For this review, take the finished solid that the model builds, in its own axes (mm). A direction names the side the tool comes from. Give positions to 0.01 mm unless a question says otherwise; leave off trailing zeros. Loops run counter-clockwise (first coordinate to the right, second up) from the corner with the lowest first, then second, coordinate; pieces in that order, holes last.
```python
from build123d import *

# Parameters (mm, degrees)
SKETCH_1_R          = 11
SKETCH_1_R_2        = 1
EXTRUDE_1_DEPTH     = 4
EXTRUDE_START       = -12
SKETCH_3_R          = 1
EXTRUDE_2_DEPTH     = 12
SKETCH_12_R         = 1
CUT_EXTRUDE_4_DEPTH = 20
SKETCH_13_R         = 7.5
CUT_EXTRUDE_5_DEPTH = 17.062378404
EXTRUDE_START_2     = -1
SKETCH_14_R         = 1
EXTRUDE_3_DEPTH     = 1
CHAMFER_1_SIZE      = 0.2


with BuildPart() as part:
    # 草图1 → 凸台-拉伸1 (new body)
    with BuildSketch(Plane.XY):
        Circle(SKETCH_1_R)
        with Locations((9, 0)):
            Circle(SKETCH_1_R_2, mode=Mode.SUBTRACT)
        with Locations((2.781152949, -8.559508647)):
            Circle(SKETCH_1_R_2, mode=Mode.SUBTRACT)
        with Locations((-7.281152949, -5.290067271)):
            Circle(SKETCH_1_R_2, mode=Mode.SUBTRACT)
        with Locations((-7.281152949, 5.290067271)):
            Circle(SKETCH_1_R_2, mode=Mode.SUBTRACT)
        with Locations((2.781152949, 8.559508647)):
            Circle(SKETCH_1_R_2, mode=Mode.SUBTRACT)
    extrude(amount=EXTRUDE_1_DEPTH)

    # 草图3 → 凸台-拉伸2 (add)
    with BuildSketch(Plane.XY.offset(4).offset(EXTRUDE_START)):
        with Locations((9, 0)):
            Circle(SKETCH_3_R)
        with Locations((2.781152949, -8.559508647)):
            Circle(SKETCH_3_R)
        with Locations((-7.281152949, -5.290067271)):
            Circle(SKETCH_3_R)
        with Locations((-7.281152949, 5.290067271)):
            Circle(SKETCH_3_R)
        with Locations((2.781152949, 8.559508647)):
            Circle(SKETCH_3_R)
    extrude(amount=EXTRUDE_2_DEPTH)

    # 草图12 → 切除-拉伸4 (cut)
    with BuildSketch(Plane(origin=(0, 0, -8), x_dir=(-1, 0, 0), z_dir=(0, 0, -1))):
        with Locations(Location((-2.781152949, -8.559508647, 0), (0, 0, 180))):
            Circle(SKETCH_12_R)
        with Locations(Location((7.281152949, 5.290067271, 0), (0, 0, 180))):
            Circle(SKETCH_12_R)
        with Locations(Location((-2.781152949, 8.559508647, 0), (0, 0, 180))):
            Circle(SKETCH_12_R)
        with Locations(Location((-9, 0, 0), (0, 0, 180))):
            Circle(SKETCH_12_R)
        with Locations(Location((7.281152949, -5.290067271, 0), (0, 0, 180))):
            Circle(SKETCH_12_R)
    extrude(amount=-CUT_EXTRUDE_4_DEPTH, mode=Mode.SUBTRACT)

    # 草图13 → 切除-拉伸5 (cut, through all)
    with BuildSketch(Plane.XY.offset(4)):
        Circle(SKETCH_13_R)
    extrude(amount=-CUT_EXTRUDE_5_DEPTH, mode=Mode.SUBTRACT)

    # 草图14 → 凸台-拉伸3 (add)
    with BuildSketch(Plane.XY.offset(4).offset(EXTRUDE_START_2)):
        with Locations((-7.281152949, -5.290067271)):
            Circle(SKETCH_14_R)
        with Locations((2.781152949, -8.559508647)):
            Circle(SKETCH_14_R)
        with Locations((9, 0)):
            Circle(SKETCH_14_R)
        with Locations((2.781152949, 8.559508647)):
            Circle(SKETCH_14_R)
        with Locations((-7.281152949, 5.290067271)):
            Circle(SKETCH_14_R)
    extrude(amount=EXTRUDE_3_DEPTH)

    # 倒角1
    chamfer_1_edges = [part.edges().sort_by_distance(p)[0] for p in [
        (-11, 0, 0),
        (-11, 0, 4),
        (-7.5, 0, 0),
        (-7.5, 0, 4),
    ]]
    chamfer(chamfer_1_edges, length=CHAMFER_1_SIZE)


solid = part.part
```
Q1. For pin 1 Ø1.6 at (x, y) = (2.78, -8.56) entering from -Z; pin 2 Ø1.5 at (y, z) = (2, 3) entering from -X; pin 3 Ø1 at (y, z) = (-3.5, 2) entering from -X, all flat-tipped, find the tip position at first contact; note any pin that passes through.
Answers:
pin 1: stops at z = 3
pin 2: stops at x = -10.93
pin 3: stops at x = -10.58
Q2. Mouldability with a two-part tool opening along Y and no side actions: class faces 1 (the flat face through (3, 9, 3)), 2 (the flat face through (6, -6, 0)), 3 (the cylindrical face through (-2.38, -10.74, 1.97)) as +Y half, -Y half, draft (parallel to the pull), parting line (faces both ways), or undercut.
Answers:
face 1: undercut
face 2: draft
face 3: parting line
Q3. Consider section B-B on x = 0. Give the boundary of the cut face in (y, z), plus the area to 3 significant figures.
Answers:
outline: (-11, 0.2) - (-10.8, 0) - (-7.7, 0) - (-7.5, 0.2) - (-7.5, 3.8) - (-7.7, 4) - (-10.8, 4) - (-11, 3.8) - close; (7.5, 0.2) - (7.7, 0) - (10.8, 0) - (11, 0.2) - (11, 3.8) - (10.8, 4) - (7.7, 4) - (7.5, 3.8) - close
area: 27.8 mm2
Q4. Consider section A-A on y = 0. Give the boundary of the cut face in (x, z), plus the area to 3 significant figures.
Answers:
outline: (-11, 0.2) - (-10.8, 0) - (-7.7, 0) - (-7.5, 0.2) - (-7.5, 3.8) - (-7.7, 4) - (-10.8, 4) - (-11, 3.8) - close; (7.5, 0.2) - (7.7, 0) - (8, 0) - (8, 3) - (10, 3) - (10, 0) - (10.8, 0) - (11, 0.2) - (11, 3.8) - (10.8, 4) - (7.7, 4) - (7.5, 3.8) - close
area: 21.8 mm2
Q5. Machinability: for faces 4 (the flat face through (5, -7, 4)), 5 (the flat face through (-7, 5, 3)), which of the approach directions +Z, -Z, +X, -X, +Y, -Y give a long, thin tool a straight path to every point of the face, cutting with its end or side? Answer none if there is none.
Answers:
face 4: +Z, +X, -X, +Y, -Y
face 5: -Z
Q6. Consider section C-C on z = 2.7. Give the boundary of the cut face in (x, y), plus the area to 3 significant figures.
Answers:
outline: circle Ø22 at (0, 0); hole circle Ø2 at (-7.28, -5.29); hole circle Ø2 at (-7.28, 5.29); hole circle Ø15 at (0, 0); hole circle Ø2 at (2.78, -8.56); hole circle Ø2 at (2.78, 8.56); hole circle Ø2 at (9, 0)
area: 188 mm2
Q7. For probe 1 along Y at (x, z) = (0, 1.1); probe 2 along Y at (x, z) = (-8, 2.6); probe 3 along X at (y, z) = (2.25, 3.5), list the stretches that pass through material, from the lowest coordinate up.
Answers:
probe 1: y = -11 to -7.5, 7.5 to 11
probe 2: y = -7.55 to -5.99, -4.59 to 4.59, 5.99 to 7.55
probe 3: x = -10.77 to -7.15, 7.15 to 10.77
